Verification items for the finished model (mm, model axes). A direction names the side the tool comes from. Coordinates: 2 decimals unless noted, no trailing zeros. Loops run counter-clockwise (first coordinate to the right, second up) from the corner with the lowest first, then second, coordinate; pieces in that order, holes last. Notation, with made-up numbers: (-32, -9) -> (-25, -9) arc R26 ccw to (-25, 21) -> close; hole circle Ø9 at (27, 13). An arc over 180 degrees is marked (long way). Answer as a JSON object with one key per item and string values. Group by question number.
Q1. Gauge pin test, flat ends, axial feed: pin 1 Ø1.8 at (y, z) = (-2.5, -1.5) entering from -X; pin 2 Ø1.5 at (y, z) = (-0.5, 35) entering from +X; pin 3 Ø6 at (x, y) = (5.5, -7) entering from -Z; pin 4 Ø2 at (x, z) = (-10, 24.5) entering from -Y. Record the tip position at first contact, or that the pin passes through.
Q2. Cross-section at D-D on y = -8. Record the boundary of the cut face in (x, z), and give its area (3 significant figures).
Q3. Set-up check for faces 1 (the cylindrical face through (-1.36, -5.58, -23.48)), 2 (the flat face through (-5, 0, 33)), 3 (the flat face through (7, -1, 13.188)): record each of +Z, -Z, +X, -X, +Y, -Y from which the full face is reachable in a straight line by a thin tool's end or side.
Q4. Release check for a two-part mould opening along Z. For faces 4 (the flat face through (-2, -4, 14)), 5 (the flat face through (0.79, -1.97, 0.58)), 6 (the flat face through (-2, 0, -19.538)), 7 (the cylindrical face through (5.37, -1.54, 21.54)) record: released by +Z, released by -Z, zero draft, split by the parting line, or undercut.
Q5. Cross-section at A-A on z = -15. Record the boundary of the cut face in (x, y), and give its area (3 significant figures).
Q6. Scan lines: L1, parallel to Z at x = 2.75, y = -4.5; L2, parallel to X at y = -0.75, z = 25; L3, parallel to Y at x = -4.75, z = -6.5. Record each from-to range of solid material in increasing order.
Q7. Cross-section at B-B on x = 9.75. Record the boundary of the cut face in (y, z).
```python
from build123d import *

# Parameters (mm, degrees)
SKETCH1_W            = 12
SKETCH1_H            = 60
BOSS_EXTRUDE1_DEPTH  = 1
SKETCH4_W            = 12
SKETCH4_H            = 60
BOSS_EXTRUDE5_DEPTH  = 4
SKETCH3_W            = 0.442585723
SKETCH3_H            = 46.400729484
SKETCH3_W_2          = 0.4
CUT_EXTRUDE1_DEPTH   = 3
BOSS_EXTRUDE6_DEPTH  = 7
BOSS_EXTRUDE11_DEPTH = 8
BOSS_EXTRUDE12_DEPTH = 2
BOSS_EXTRUDE13_DEPTH = 0.75
BOSS_EXTRUDE15_DEPTH = 2
BOSS_EXTRUDE16_DEPTH = 5
FILLET1_R            = 2.5
FILLET2_R            = 2.5


with BuildPart() as part:
    # Sketch1 → Boss-Extrude1 (new body)
    with BuildSketch(Plane(origin=(0, 0, 0), x_dir=(1, 0, 0), z_dir=(0, 1, 0))):
        with Locations((-1.342029662, -10.461538462)):
            Rectangle(SKETCH1_W, SKETCH1_H)
    extrude(amount=BOSS_EXTRUDE1_DEPTH)

    # Sketch4 → Boss-Extrude5 (add)
    with BuildSketch(Plane(origin=(0, 0, 0), x_dir=(1, 0, 0), z_dir=(0, 1, 0))):
        with Locations((-1.342029662, -10.461538462)):
            Rectangle(SKETCH4_W, SKETCH4_H)
        Polygon((-2.096130055, -33.457130572), (-6.384615385, -37.75443168), (-6.384611455, -29.168649172), align=None, mode=Mode.SUBTRACT)
        Polygon((2.908277834, -38.461538462), (-5.677508603, -38.461538462), (-1.384615385, -34.168645243), align=None, mode=Mode.SUBTRACT)
        Polygon((-1.38975443, -32.749302861), (-5.677336591, -28.461186458), (-1.384615385, -24.168121227), (2.898997747, -28.451734358), align=None, mode=Mode.SUBTRACT)
        Polygon((-2.091498793, -23.461237818), (-6.384610808, -27.754427103), (-6.384606877, -19.168129734), align=None, mode=Mode.SUBTRACT)
        Polygon((-1.384401984, -22.754128282), (-5.676963509, -18.461572954), (-1.384618257, -14.16814285), (2.90844487, -18.461204162), align=None, mode=Mode.SUBTRACT)
        Polygon((-2.094846949, -13.457914458), (-6.38460623, -17.742175237), (-6.38460623, -9.168156991), align=None, mode=Mode.SUBTRACT)
        Polygon((3.615384615, -29.168645243), (3.615384615, -37.75443168), (-0.749170508, -33.533200366), align=None, mode=Mode.SUBTRACT)
        Polygon((3.615384615, -19.168465252), (3.615384615, -27.753907665), (-0.677336591, -23.461186458), align=None, mode=Mode.SUBTRACT)
        Polygon((3.615384615, -17.754251693), (-0.676897524, -13.461506969), (3.615384615, -9.169224829), align=None, mode=Mode.SUBTRACT)
        Polygon((-6.384597723, 0.832144172), (-2.091409836, -3.461043715), (-6.384601653, -7.753916614), align=None, mode=Mode.SUBTRACT)
        Polygon((2.908517821, -8.460971372), (-1.387204346, -12.751178894), (-5.677010576, -8.461229413), (-1.384615385, -4.167838166), align=None, mode=Mode.SUBTRACT)
        Polygon((-1.385221722, -2.75490806), (-5.679497842, 1.537745361), (-1.38541394, 5.831829263), (2.908210299, 1.538205024), align=None, mode=Mode.SUBTRACT)
        Polygon((-2.089578329, 6.535993652), (-6.3837953, 2.241776681), (-6.384597078, 2.240974904), (-6.384597078, 2.242578156), (-6.384593146, 10.83100847), align=None, mode=Mode.SUBTRACT)
        Polygon((-5.677832652, 11.538461538), (2.912889557, 11.538461538), (-1.382471548, 7.243100433), align=None, mode=Mode.SUBTRACT)
        Polygon((3.615384615, -7.755011267), (-0.677821818, -3.462040655), (3.615384615, 0.831165778), align=None, mode=Mode.SUBTRACT)
        Polygon((3.615384615, 2.245379341), (-0.678307159, 6.538936044), (3.615384615, 10.832627818), align=None, mode=Mode.SUBTRACT)
    extrude(amount=-BOSS_EXTRUDE5_DEPTH)

    # Sketch3 → Cut-Extrude1 (cut)
    with BuildSketch(Plane.XZ.offset(4)):
        with Locations((3.436677476, 13.26117372)):
            Rectangle(SKETCH3_W, SKETCH3_H)
        with Locations((-6.184615385, 13.26117372)):
            Rectangle(SKETCH3_W_2, SKETCH3_H)
    extrude(amount=-CUT_EXTRUDE1_DEPTH, mode=Mode.SUBTRACT)

    # Sketch5 → Boss-Extrude6 (add)
    with BuildSketch(Plane(origin=(0, 0, -19.538461538), x_dir=(-1, 0, 0), z_dir=(0, 0, -1))):
        Polygon((-12.288789064, 5.355892869), (14.972848388, 5.355892869), (3.537352374, -9.415920613), (1.425918842, -12.033387248), (-0.689767913, -9.409188123), align=None)
        with BuildLine():
            Line((9.692725832, 1.966121199), (9.999443939, 1.857726092))
            Line((9.999443939, 1.857726092), (10.306162047, 1.966121199))
            ThreePointArc((10.306162047, 1.966121199), (9.999443939, 3.917921599), (9.692725832, 1.966121199))
        make_face(mode=Mode.SUBTRACT)
        with BuildLine():
            Line((-7.622102723, 1.966121199), (-7.315384615, 1.857726092))
            Line((-7.315384615, 1.857726092), (-7.008666508, 1.966121199))
            ThreePointArc((-7.008666508, 1.966121199), (-7.315384615, 3.917921599), (-7.622102723, 1.966121199))
        make_face(mode=Mode.SUBTRACT)
        with BuildLine():
            Line((0.921478569, 1.79402802), (1.342029662, 1.636661499))
            Line((1.342029662, 1.636661499), (1.762580755, 1.79402802))
            ThreePointArc((1.762580755, 1.79402802), (1.342029662, 4.117921599), (0.921478569, 1.79402802))
        make_face(mode=Mode.SUBTRACT)
    extrude(amount=-BOSS_EXTRUDE6_DEPTH)

    # Sketch5<3> → Boss-Extrude11 (add)
    with BuildSketch(Plane(origin=(0, 0, -19.538461538), x_dir=(-1, 0, 0), z_dir=(0, 0, -1))):
        with BuildLine():
            Line((3.537352374, -9.415920613), (1.425918842, -12.033387248))
            Line((1.425918842, -12.033387248), (-0.689767913, -9.409188123))
            ThreePointArc((-0.689767913, -9.409188123), (1.429900561, -5.57732435), (3.537352374, -9.415920613))
        make_face()
    extrude(amount=BOSS_EXTRUDE11_DEPTH)

    # Sketch11 → Boss-Extrude12 (add)
    with BuildSketch(Plane.ZY.offset(7.342029662)):
        Polygon((-12.538461538, 5.355892869), (-4.993833778, 1), (-12.538461538, 1), align=None)
    extrude(amount=-BOSS_EXTRUDE12_DEPTH)

    # Sketch12 → Boss-Extrude13 (add, symmetric)
    with BuildSketch(Plane.ZY.offset(1.342029662)):
        Polygon((-13.859142787, 0.316720052), (-13.859142787, -4.418628297), (-13.859142787, -9.68323793), (-6.410996577, -3.888931374), (-6.410996577, 0.316720052), align=None)
    extrude(amount=BOSS_EXTRUDE13_DEPTH, both=True)

    # Sketch14 → Boss-Extrude15 (add)
    with BuildSketch(Plane(origin=(4.657970338, 0, 0), x_dir=(0, 0, -1), z_dir=(1, 0, 0))):
        Polygon((4.993833778, 1), (12.538461538, 5.355892869), (12.538461538, 1), align=None)
    extrude(amount=-BOSS_EXTRUDE15_DEPTH)

    # Sketch15 → Boss-Extrude16 (add)
    with BuildSketch(Plane(origin=(0, 1, 0), x_dir=(1, 0, 0), z_dir=(0, 1, 0))):
        Polygon((4.657970338, -11.687539089), (4.657970338, -13.187539089), (8.957970338, -13.187539089), (8.957970338, -19.287539089), (4.657970338, -19.287539089), (4.657970338, -20.787539089), (10.457970338, -20.787539089), (10.457970338, -11.687539089), align=None)
    extrude(amount=-BOSS_EXTRUDE16_DEPTH)

    # Fillet1
    fillet1_edges = [part.edges().sort_by_distance(p)[0] for p in [
        (4.657970338, -1.5, 20.787539089),
    ]]
    fillet(fillet1_edges, radius=FILLET1_R)

    # Fillet2
    fillet2_edges = [part.edges().sort_by_distance(p)[0] for p in [
        (4.657970338, -1.5, 11.687539089),
    ]]
    fillet(fillet2_edges, radius=FILLET2_R)


solid = part.part
```
Computed values:
{
 "1": {"pin 1": "stops at x = -7.34", "pin 2": "stops at x = 4.66", "pin 3": "stops at z = -19.54", "pin 4": "passes through"},
 "2": {"outline": "(-4.63, -19.54) -> (-3.92, -19.54) -> (-3.92, -27.54) -> (1.07, -27.54) -> (1.07, -19.54) -> (1.8, -19.54) -> (1.8, -12.54) -> (-0.59, -12.54) -> (-0.59, -11.7) -> (-2.09, -11.7) -> (-2.09, -12.54) -> (-4.63, -12.54) -> close", "area": "86.3 mm²"},
 "3": {"face 1": "-Z", "face 2": "-Y", "face 3": "+Y, -Y"},
 "4": {"face 4": "zero draft", "face 5": "undercut", "face 6": "released by -Z", "face 7": "released by +Z"},
 "5": {"outline": "(-14.97, 5.36) -> (-3.54, -9.42) -> (-1.43, -12.03) -> (0.69, -9.41) -> (12.29, 5.36) -> close; hole (-10.31, 1.97) -> (-10, 1.86) -> (-9.69, 1.97) arc R1 ccw (long way) to start; hole (-1.76, 1.79) -> (-1.34, 1.64) -> (-0.92, 1.79) arc R1.2 ccw (long way) to start; hole (7.01, 1.97) -> (7.32, 1.86) -> (7.62, 1.97) arc R1 ccw (long way) to start", "area": "227 mm²"},
 "6": {"L1": "z = -19.54 to -12.54", "L2": "x = -7.34 to -6.38, -3.63 to -2.22, -0.55 to 0.86, 3.62 to 4.66", "L3": "y = 0 to 1"},
 "7": {"outline": "(-4, 11.69) -> (1, 11.69) -> (1, 20.79) -> (-4, 20.79) -> close; (2.12, -19.54) -> (5.36, -19.54) -> (5.36, -12.54) -> (2.12, -12.54) -> close"}
}
